```python
from build123d import *

# Parameters (mm, degrees)
BOSS_EXTRUDE1_DEPTH = 98.425
CUT_EXTRUDE2_DEPTH  = 98.425
SKETCH5_R           = 1.651
CUT_EXTRUDE3_DEPTH  = 13.5992
FILLET1_R           = 2.54
SKETCH6_R           = 1.651
CUT_EXTRUDE4_DEPTH  = 98.425


with BuildPart() as part:
    # Sketch1 → Boss-Extrude1 (new body)
    with BuildSketch(Plane(origin=(0, 0, 0), x_dir=(0, 0, -1), z_dir=(1, 0, 0))):
        with BuildLine():
            Line((0, 16.7996), (0, 3.2004))
            Line((0, 3.2004), (9.525, 3.2004))
            Line((9.525, 3.2004), (9.525, 0))
            Line((9.525, 0), (14.605, 0))
            ThreePointArc((14.605, 0), (15.279774052, 1.174548121), (15.868724182, 2.394392806))
            Line((15.868724182, 2.394392806), (23.603930172, 20))
            Line((23.603930172, 20), (9.525, 20))
            Line((9.525, 20), (9.525, 16.7996))
            Line((9.525, 16.7996), (0, 16.7996))
        make_face()
    extrude(amount=BOSS_EXTRUDE1_DEPTH)

    # Sketch4 → Cut-Extrude2 (cut)
    with BuildSketch(Plane.ZY):
        with BuildLine():
            Line((0, 13.526281186), (0, 6.473718814))
            ThreePointArc((0, 6.473718814), (-2.36728, 10), (0, 13.526281186))
        make_face()
    extrude(amount=-CUT_EXTRUDE2_DEPTH, mode=Mode.SUBTRACT)

    # Sketch5 → Cut-Extrude3 (cut)
    with BuildSketch(Plane(origin=(0, 16.7996, 0), x_dir=(1, 0, 0), z_dir=(0, 1, 0))):
        with Locations((17.4625, 4.7625)):
            Circle(SKETCH5_R)
        with Locations((80.9625, 4.7625)):
            Circle(SKETCH5_R)
    extrude(amount=-CUT_EXTRUDE3_DEPTH, mode=Mode.SUBTRACT)

    # Fillet1
    fillet1_edges = [part.edges().sort_by_distance(p)[0] for p in [
        (49.2125, 20, -23.603930172),
        (49.2125, 0, -14.605),
    ]]
    fillet(fillet1_edges, radius=FILLET1_R)

    # Sketch6 → Cut-Extrude4 (cut)
    with BuildSketch(Plane(origin=(98.425, 0, 0), x_dir=(0, 0, -1), z_dir=(1, 0, 0))):
        with Locations((9.525, 10)):
            Circle(SKETCH6_R)
    extrude(amount=-CUT_EXTRUDE4_DEPTH, mode=Mode.SUBTRACT)


solid = part.part
```
Could you check a few things on this model? Use its own coordinates, in mm. A direction names the side the tool comes from. Give positions to 0.01 mm unless a question says otherwise; leave off trailing zeros. Order: outer loops, then holes, each group sorted by start corner. A loop starts at its lowest first (then second) coordinate and runs counter-clockwise, first axis right, second up.
Q1. We'd pull the mould along Y, two halves only. Please class faces 4 (the flat face through (49, 15, 0)), 5 (the cylindrical face through (49.901, 0.383, -14.469)), 6 (the cylindrical face through (49.9, 9, -8.21)): +Y half, -Y half, draft (parallel to the pull), parting line (faces both ways), or undercut.
Q2. Suppose I cut it at B-B, the plane x = 65. Write out the boundary of the cut face in (y, z) (3 decimals).
Q3. If I drill on line 1 along X through (y, z) = (15, -3.5) (3 decimals); line 2 along Y through (x, z) = (15, -7.5); line 3 along Y through (x, z) = (48, -8.75), over which ranges is the centre line in solid material (lowest first)?
Q4. Suppose I cut it at A-A, the plane y = 10. Write out the boundary of the cut face in (x, z) (1 decimal), and give its area (3 significant figures).
Q5. Suppose I cut it at C-C, the plane y = 4.25. Write out the boundary of the cut face in (x, z) (1 decimal).
Q6. Suppose I cut it at D-D, the plane z = -17. Write out the boundary of the cut face in (x, y) (3 decimals), and give its area (3 significant figures).
Q7. I'm going to push flat-ended pins straight in: P1, Ø10, axis at x = 62.5, z = -12.5, coming from the -Y side; P2, Ø3, axis at x = 56, z = -17.5, coming from the -Y side; P3, Ø10.5, axis at x = 46, z = -2.5, coming from the -Y side; P4, Ø1.6, axis at x = 65, y = 2, coming from the +Z side (3 decimals). Where does each tip first touch, or does it pass through?
Q8. For faces 1 (the flat face through (49, 2, -9.525)), 2 (the flat face through (49, 16.8, -5)), 3 (the flat face through (98.425, 12, -11)), which set-ups out of +Z, -Z, +X, -X, +Y, -Y let a thin tool reach every point of the face, with its end or its side?
Solution:
1. face 4: draft
1. face 5: -Y half
1. face 6: undercut
2. outline: (0, -13.127) arc R2.54 ccw to (1.382, -15.388) arc R18.908 ccw to (2.394, -15.869) - (16.438, -22.039) arc R2.54 ccw to (20, -19.714) - (20, -9.525) - (16.8, -9.525) - (16.8, 0) - (13.526, 0) arc R3.81 cw to (6.474, 0) - (3.2, 0) - (3.2, -9.525) - (0, -9.525) - close; hole circle Ø3.302 at (10, -9.525)
3. line 1: x = 0 to 16.399, 18.526 to 79.899, 82.026 to 98.425
3. line 2: y = 3.2 to 16.8
3. line 3: y = 3.2 to 8.54, 11.46 to 16.8
4. outline: (0, -19.2) - (98.4, -19.2) - (98.4, -11.2) - (0, -11.2) - close; (0, -7.9) - (98.4, -7.9) - (98.4, -2.4) - (0, -2.4) - close; hole circle Ø3.3 at (17.5, -4.8); hole circle Ø3.3 at (81, -4.8)
4. area: 1,320 mm2
5. outline: (0, -16.7) - (98.4, -16.7) - (98.4, 0) - (0, 0) - close; hole circle Ø3.3 at (17.5, -4.8); hole circle Ø3.3 at (81, -4.8)
6. outline: (0, 4.969) - (98.425, 4.969) - (98.425, 20) - (0, 20) - close
6. area: 1,480 mm2
7. P1: stops at y = 0
7. P2: stops at y = 2.69
7. P3: stops at y = 3.2
7. P4: stops at z = -9.525
8. face 1: +Z, +X, -X, -Y
8. face 2: +Z, +X, -X, +Y
8. face 3: +Z, -Z, +X, +Y, -Y
